Read the model definition and answer for the solid it produces. Units are mm, in the model's axes. A direction names the side the tool comes from. Give positions to 0.01 mm unless a question says otherwise; leave off trailing zeros. Order: outer loops, then holes, each group sorted by start corner. A loop starts at its lowest first (then second) coordinate and runs counter-clockwise, first axis right, second up. Notation, with made-up numbers: (44, 47) - (90, 47) arc R19 cw to (90, 62) - close; hole circle Ø3 at (77, 86). An arc over 180 degrees is marked (long way). Use a Markdown table: item, result. Add a question column.
1. A flat-ended cylindrical pin translates along its axis: P1, Ø6, axis at x = -10.52, z = -9.27, coming from the +Y side. Find the tip coordinate at first contact, or state that the pin passes through.
2. A cutting plane is placed at D-D on y = 4.25. State how many separate pieces and enclosed holes the cut face has, and give its area (3 significant figures).
3. A cutting plane is placed at A-A on x = 40.5. Determine the outline of the cut face in (y, z), and give its area (4 significant figures).
4. A cutting plane is placed at B-B on z = -0.5. Determine the outline of the cut face in (x, y).
5. For a pull along Z with two mould halves and no side action, classify faces 1 (the flat face through (38.499, 3, -9)), 2 (the flat face through (7, 3, -35.942)), 3 (the flat face through (-55.227, 3, -9)), 4 (the flat face through (7, 3, 17.398)) as released by +Z, released by -Z, zero draft, split by the parting line, or undercut.
6. Consider L1, parallel to X at y = 3.75, z = -20; L2, parallel to Z at x = 48.5, y = 4.5; L3, parallel to X at y = 2.25, z = 6.5. Determine where each line is inside the solid, lowest interval first.
7. A cutting plane is placed at C-C on z = -7.5. Determine the outline of the cut face in (x, y).
8. Which of the six approach directions +Z, -Z, +X, -X, +Y, -Y give full straight-line access (tool end or side, diameter ignored) to faces 5 (the flat face through (-7, 6.35, -10)), 6 (the flat face through (-35.923, 3, -9))?
```python
from build123d import *

# Parameters (mm, degrees)
SKETCH1_W           = 127
SKETCH1_H           = 53.34
SKETCH1_R           = 3.302
SKETCH1_W_2         = 13.97
SKETCH1_H_2         = 37.592
SKETCH1_W_3         = 14.732
BOSS_EXTRUDE1_DEPTH = 6.35


with BuildPart() as part:
    # Sketch1 → Boss-Extrude1 (new body)
    with BuildSketch(Plane(origin=(0, 0, 0), x_dir=(1, 0, 0), z_dir=(0, 1, 0))):
        with Locations((8.27250506, 9.271742923)):
            Rectangle(SKETCH1_W, SKETCH1_H)
        with Locations((-45.57549494, -9.524257077)):
            Circle(SKETCH1_R, mode=Mode.SUBTRACT)
        with Locations((-45.57549494, 28.067742923)):
            Circle(SKETCH1_R, mode=Mode.SUBTRACT)
        with Locations((62.12050506, -9.524257077)):
            Circle(SKETCH1_R, mode=Mode.SUBTRACT)
        with Locations((62.12050506, 28.067742923)):
            Circle(SKETCH1_R, mode=Mode.SUBTRACT)
        with Locations((-10.52349494, 9.271742923)):
            Circle(SKETCH1_R, mode=Mode.SUBTRACT)
        with Locations((27.06850506, 9.271742923)):
            Circle(SKETCH1_R, mode=Mode.SUBTRACT)
        with Locations((-28.93849494, 9.271742923)):
            Rectangle(SKETCH1_W_2, SKETCH1_H_2, mode=Mode.SUBTRACT)
        with Locations((45.48350506, 9.271742923)):
            Rectangle(SKETCH1_W_2, SKETCH1_H_2, mode=Mode.SUBTRACT)
        with Locations((8.27250506, 9.271742923)):
            Rectangle(SKETCH1_W_3, SKETCH1_H_2, mode=Mode.SUBTRACT)
    extrude(amount=BOSS_EXTRUDE1_DEPTH)


solid = part.part
```
Output values:
| question | item | result |
|---|---|---|
| 1 | P1 | through |
| 2 | separate pieces | 1 |
| 2 | enclosed holes | 9 |
| 2 | area | 4,960 mm² |
| 3 | outline | (0, -35.94) - (6.35, -35.94) - (6.35, -28.07) - (0, -28.07) - close; (0, 9.52) - (6.35, 9.52) - (6.35, 17.4) - (0, 17.4) - close |
| 3 | area | 100.0 mm² |
| 4 | outline | (-55.23, 0) - (-35.92, 0) - (-35.92, 6.35) - (-55.23, 6.35) - close; (-21.95, 0) - (0.91, 0) - (0.91, 6.35) - (-21.95, 6.35) - close; (15.64, 0) - (38.5, 0) - (38.5, 6.35) - (15.64, 6.35) - close; (52.47, 0) - (71.77, 0) - (71.77, 6.35) - (52.47, 6.35) - close |
| 5 | face 1 | undercut |
| 5 | face 2 | released by -Z |
| 5 | face 3 | zero draft |
| 5 | face 4 | released by +Z |
| 6 | L1 | -55.23 to -35.92, -21.95 to 0.91, 15.64 to 38.5, 52.47 to 71.77 |
| 6 | L2 | -35.94 to -28.07, 9.52 to 17.4 |
| 6 | L3 | -55.23 to -46.9, -44.25 to -35.92, -21.95 to 0.91, 15.64 to 38.5, 52.47 to 60.79, 63.45 to 71.77 |
| 7 | outline | (-55.23, 0) - (-35.92, 0) - (-35.92, 6.35) - (-55.23, 6.35) - close; (-21.95, 0) - (-13.31, 0) - (-13.31, 6.35) - (-21.95, 6.35) - close; (-7.74, 0) - (0.91, 0) - (0.91, 6.35) - (-7.74, 6.35) - close; (15.64, 0) - (24.28, 0) - (24.28, 6.35) - (15.64, 6.35) - close; (29.85, 0) - (38.5, 0) - (38.5, 6.35) - (29.85, 6.35) - close; (52.47, 0) - (71.77, 0) - (71.77, 6.35) - (52.47, 6.35) - close |
| 8 | face 5 | +Z, -Z, +X, -X, +Y |
| 8 | face 6 | +Y, -Y |
